Part model, mm, in its own coordinate system. A direction names the side the tool comes from. Coordinates: 2 decimals unless noted, no trailing zeros. Order: outer loops, then holes, each group sorted by start corner. A loop starts at its lowest first (then second) coordinate and runs counter-clockwise, first axis right, second up. Notation, with made-up numbers: (-11, -31.75) - (7, -31.75) arc R9 ccw to (7, -19.75) - close; hole circle Ø8 at (84, 80.25). An arc over 180 degrees is marked (long way). Use a Markdown table: item, result. Add a question column.
1) Two-plate mould, pull along X, no slides. Class faces 1 (the face through (-6.604, 6, 6)), 2 (the face through (28.49, -8.28, 6.26)), 3 (the face through (0, 0, 12.7)), 4 (the face through (-7.314, 3.75, 6.261)): +X half, -X half, draft (parallel to the pull), parting line (faces both ways), or undercut.
2) Tool access for faces 5 (the face through (8.022, -8.706, 6.261)), 6 (the face through (0, 8.128, 6)), 7 (the face through (18, 9.048, 6)): list every direction of +Z, -Z, +X, -X, +Y, -Y with a clear straight run to the whole face (end or side of a thin tool).
3) Saw through at C-C on x = -5. List the corners of the cut face in (y, z), then the cut area to 3 significant figures.
4) Drop a flat-ended pin along its axis: P1, Ø6.5, axis at x = 1.5, z = 7, coming from the -Y side. Give the stop position or say it passes through.
5) Saw through at B-B on z = 4.25. List the corners of the cut face in (x, y) (3 decimals).
6) Saw through at A-A on y = 6. List the corners of the cut face in (x, z), then the cut area to 3 significant figures.
7) Wall check: L1, parallel to X at y = 4, z = 5; L2, parallel to X at y = -7.25, z = 9.25; L3, parallel to Y at x = -5.5, z = 2.25. Give the ranges that are in metal, low to high. Write a range as [from, to].
Autodesk Inventor part; units mm, degrees
ref_plane "YZ Plane" through (0, 0, 0) normal (1, 0, 0) x (0, 1, 0)
ref_plane "XZ Plane" through (0, 0, 0) normal (0, 1, 0) x (-1, 0, 0)
ref_plane "XY Plane" through (0, 0, 0) normal (0, 0, 1) x (1, 0, 0)
sketch "Sketch1" plane through (0, 0, 0) normal (0, 0, 1) x (1, 0, 0)
  line L0 (0, 8.128) -> (-6.604, 8.128)
  line L1 (-6.604, 8.128) -> (-6.604, 3.4598)
  arc A0 (-7.62, 4.4758) -> (-6.604, 3.4598) centre (-6.604, 4.4758) ccw
  line L2 (-7.62, 4.4758) -> (-7.62, 7.779)
  line L3 (-29.21, 6.5078) -> (-29.21, 0)
  arc A1 (-7.62, 7.779) -> (-8.945, 9.0478) centre (-8.89, 7.779) ccw
  line L4 (-8.945, 9.0478) -> (-26.67, 9.0478)
  arc A2 (-26.67, 9.0478) -> (-29.21, 6.5078) centre (-26.67, 6.5078) ccw
  line L5 (0, 8.128) -> (6.604, 8.128)
  line L6 (6.604, 8.128) -> (6.604, 3.4598)
  arc A3 (6.604, 3.4598) -> (7.62, 4.4758) centre (6.604, 4.4758) ccw
  line L7 (7.62, 4.4758) -> (7.62, 7.779)
  line L8 (29.21, 6.5078) -> (29.21, 0)
  arc A4 (8.945, 9.0478) -> (7.62, 7.779) centre (8.89, 7.779) ccw
  line L9 (8.945, 9.0478) -> (26.67, 9.0478)
  arc A5 (29.21, 6.5078) -> (26.67, 9.0478) centre (26.67, 6.5078) ccw
  line L10 (0, -8.128) -> (-6.604, -8.128)
  line L11 (-6.604, -8.128) -> (-6.604, -3.4598)
  arc A6 (-6.604, -3.4598) -> (-7.62, -4.4758) centre (-6.604, -4.4758) ccw
  line L12 (-7.62, -4.4758) -> (-7.62, -7.779)
  line L13 (-29.21, -6.5078) -> (-29.21, 0)
  arc A7 (-8.945, -9.0478) -> (-7.62, -7.779) centre (-8.89, -7.779) ccw
  line L14 (-8.945, -9.0478) -> (-26.67, -9.0478)
  arc A8 (-29.21, -6.5078) -> (-26.67, -9.0478) centre (-26.67, -6.5078) ccw
  line L15 (0, -8.128) -> (6.604, -8.128)
  line L16 (6.604, -8.128) -> (6.604, -3.4598)
  arc A9 (7.62, -4.4758) -> (6.604, -3.4598) centre (6.604, -4.4758) ccw
  line L17 (7.62, -4.4758) -> (7.62, -7.779)
  line L18 (29.21, -6.5078) -> (29.21, 0)
  arc A10 (7.62, -7.779) -> (8.945, -9.0478) centre (8.89, -7.779) ccw
  line L19 (8.945, -9.0478) -> (26.67, -9.0478)
  arc A11 (26.67, -9.0478) -> (29.21, -6.5078) centre (26.67, -6.5078) ccw
  point P0 (0, 0)
  dimension "d0" = 8.128
  dimension "d2" = 29.21
  dimension "d4" = 1.016
  dimension "d5" = 1.016
  dimension "d10" = 1.27
  dimension "d11" = 2.54
  dimension "d12" = 5.588
extrude "Extrusion1" add sketch "Sketch1" along normal blind 12.7
properties part number "ConnectorDE" material "ABS Plastic"
Results are:
| question | item | result |
|---|---|---|
| 1 | face 1 | undercut |
| 1 | face 2 | +X half |
| 1 | face 3 | draft |
| 1 | face 4 | undercut |
| 2 | face 5 | +Z, -Z, -Y |
| 2 | face 6 | +Z, -Z, +Y |
| 2 | face 7 | +Z, -Z, +X, -X, +Y |
| 3 | outline | (-8.13, 0) - (8.13, 0) - (8.13, 12.7) - (-8.13, 12.7) - close |
| 3 | area | 206 mm2 |
| 4 | P1 | y = -8.13 |
| 5 | outline | (-29.21, -6.508) arc R2.54 ccw to (-26.67, -9.048) - (-8.945, -9.048) arc R1.27 ccw to (-7.62, -7.779) - (-7.62, -4.476) arc R1.016 cw to (-6.604, -3.46) - (-6.604, -8.128) - (6.604, -8.128) - (6.604, -3.46) arc R1.016 cw to (7.62, -4.476) - (7.62, -7.779) arc R1.27 ccw to (8.945, -9.048) - (26.67, -9.048) arc R2.54 ccw to (29.21, -6.508) - (29.21, 6.508) arc R2.54 ccw to (26.67, 9.048) - (8.945, 9.048) arc R1.27 ccw to (7.62, 7.779) - (7.62, 4.476) arc R1.016 cw to (6.604, 3.46) - (6.604, 8.128) - (-6.604, 8.128) - (-6.604, 3.46) arc R1.016 cw to (-7.62, 4.476) - (-7.62, 7.779) arc R1.27 ccw to (-8.945, 9.048) - (-26.67, 9.048) arc R2.54 ccw to (-29.21, 6.508) - close |
| 6 | outline | (-29.21, 0) - (-7.62, 0) - (-7.62, 12.7) - (-29.21, 12.7) - close; (-6.6, 0) - (6.6, 0) - (6.6, 12.7) - (-6.6, 12.7) - close; (7.62, 0) - (29.21, 0) - (29.21, 12.7) - (7.62, 12.7) - close |
| 6 | area | 716 mm2 |
| 7 | L1 | [-29.21, -7.5], [-6.6, 6.6], [7.5, 29.21] |
| 7 | L2 | [-29.1, -7.62], [-6.6, 6.6], [7.62, 29.1] |
| 7 | L3 | [-8.13, 8.13] |
